Build history of the part. All positions in model axes, mm. A direction names the side the tool comes from. Give positions to 0.01 mm unless a question says otherwise; leave off trailing zeros. Loops run counter-clockwise (first coordinate to the right, second up) from the corner with the lowest first, then second, coordinate; pieces in that order, holes last. Notation, with made-up numbers: (-10.5, 24) -> (22.5, 24) arc R23 cw to (22.5, 49) -> close; hole circle Ø8 at (27.25, 37). An arc over 180 degrees is marked (long way). One line per question, with ' | ' between items. Start each with the question number.
(1) Mould opens along Y. For faces 3 (the face through (671, 731, 1)), 4 (the face through (363, 1947, -1)), 5 (the face through (716, 960, -1)) say: pulls with the +Y half, pulls with the -Y half, needs draft (parallel to the pull), parting line crosses it, or undercut.
(2) Slice it at B-B, the plane z = -25. Write the cut outline in (x, y).
(3) Slice it at C-C, the plane y = 1552. Write the cut outline in (x, z).
(4) Slice it at A-A, the plane x = 570.5. Write the cut outline in (y, z), then the cut area to 3 significant figures.
(5) Drill centre lines: L1, parallel to X at y = 841, z = -3; L2, parallel to Y at x = 456, z = 1.5; L3, parallel to X at y = 1561, z = -17. Where is each one in solid material? Low to high. Write a range as from..to.
(6) 3-axis set-ups, long thin cutter, end or side, ignore diameter. For faces 1 (the face through (651, 681, 1)), 2 (the face through (353, 771, -65)): which of +Z, -Z, +X, -X, +Y, -Y reach the whole face in a straight line?
Autodesk Inventor part; units mm, degrees
ref_plane "YZ Plane" through (0, 0, 0) normal (1, 0, 0) x (0, 1, 0)
ref_plane "XZ Plane" through (0, 0, 0) normal (0, 1, 0) x (-1, 0, 0)
ref_plane "XY Plane" through (0, 0, 0) normal (0, 0, 1) x (1, 0, 0)
sketch "Sketch6" plane through (0, 0, 0) normal (0, 0, 1) x (1, 0, 0)
  line L0 (0, 0) -> (716, 0)
  line L1 (716, 0) -> (716, 1947)
  line L2 (716, 1947) -> (0, 1947)
  line L3 (0, 1947) -> (0, 0)
  dimension "d0" = 716
  dimension "d1" = 1947
extrude "Extrusion1" add sketch "Sketch6" along normal mid plane 130
sketch "Sketch7" plane through (0, 0, 65) normal (0, 0, 1) x (1, 0, 0)
  circle A0 centre (358, 1447) radius 300
  line L0 (716, 1947) -> (0, 1947)
  point P0 (0, 0)
  point P1 (358, 1947)
  dimension "d4" = 600
  dimension "d5" = 500
extrude "Extrusion2" cut sketch "Sketch7" against normal up to surface (130 mm away)
sketch "Sketch9" plane through (0, 0, 65) normal (0, 0, 1) x (1, 0, 0)
  line L0 (651, 761) -> (651, 701) construction
  line L1 (671, 761) -> (671, 701)
  line L2 (631, 701) -> (631, 761)
  arc A0 (671, 761) -> (631, 761) centre (651, 761) ccw
  arc A1 (631, 701) -> (671, 701) centre (651, 701) ccw
  line L3 (0, 0) -> (716, 0)
  line L4 (0, 1947) -> (0, 0)
  circle A2 centre (651, 841) radius 3.5
  circle A3 centre (651, 654) radius 3.5
  line L5 (716, 0) -> (716, 1947)
  point P0 (651, 731)
  point P1 (651, 681)
  point P2 (651, 781)
  dimension "d8" = 40
  dimension "d9" = 681
  dimension "d10" = 100
  dimension "d12" = 7
  dimension "d13" = 60
  dimension "d14" = 7
  dimension "d15" = 187
  dimension "d18" = 65
extrude "Extrusion3" cut sketch "Sketch9" against normal up to surface (130 mm away)
equation "\"d0\" = SchuBrei"
equation "\"d1\" = SchuHoeh"
equation "\"d2\" = SchuDick"
equation "\"SchuDick\" = 130"
equation "\"SchuBrei\" = 716"
equation "\"SchuHoeh\" = 1947"
properties part number "Schutz"
Final values:
1) face 3: undercut | face 4: pulls with the +Y half | face 5: needs draft
2) outline: (0, 0) -> (716, 0) -> (716, 1947) -> (0, 1947) -> close; hole circle Ø600 at (358, 1447); hole (631, 701) arc R20 ccw to (671, 701) -> (671, 761) arc R20 ccw to (631, 761) -> close; hole circle Ø7 at (651, 654); hole circle Ø7 at (651, 841)
3) outline: (0, -65) -> (76.98, -65) -> (76.98, 65) -> (0, 65) -> close; (639.02, -65) -> (716, -65) -> (716, 65) -> (639.02, 65) -> close
4) outline: (0, -65) -> (1235.24, -65) -> (1235.24, 65) -> (0, 65) -> close; (1658.76, -65) -> (1947, -65) -> (1947, 65) -> (1658.76, 65) -> close | area: 198,000 mm2
5) L1: 0..647.5, 654.5..716 | L2: 0..1163.46, 1730.54..1947 | L3: 0..80.5, 635.5..716
6) face 1: +Z, -Z | face 2: -Z, +X, -X, +Y, -Y
